CAD build for the part. Positions are in the model's coordinates, mm. Face numbers are marked on the shaded views. Give positions to 0.01 mm unless a question says otherwise; leave off trailing zeros. Loops run counter-clockwise (first coordinate to the right, second up) from the corner with the lowest first, then second, coordinate; pieces in that order, holes last. Notation, with made-up numbers: M -27,-1 L -21,-1 A25 ccw -21,38 Z; hole C -5.5,17.5 d6. An arc over 180 degrees is marked long. Answer as CSV lines item,"result".
```python
from build123d import *

# Parameters (mm, degrees)
F0_R     = 14.235704
F0_R_2   = 10.13824
F1_DEPTH = 50.8
F2_DEPTH = 114.046


with BuildPart() as f1:
    # F0 (on Top) → F1 (new body)
    with BuildSketch(Plane.XY):
        Circle(F0_R)
        with Locations((53.975, 0)):
            Circle(F0_R_2)
        with BuildLine():
            Line((57.191927, 18.776418), (9.512184, 26.945296))
            Line((9.512184, 26.945296), (0, 28.575))
            ThreePointArc((0, 28.575), (-28.575, 0), (0, -28.575))
            Line((0, -28.575), (9.512184, -26.945296))
            Line((9.512184, -26.945296), (57.191927, -18.776418))
            ThreePointArc((57.191927, -18.776418), (73.025, 0), (57.191927, 18.776418))
        make_face()
        Circle(F0_R, mode=Mode.SUBTRACT)
        with Locations((53.975, 0)):
            Circle(F0_R_2, mode=Mode.SUBTRACT)
        with BuildLine():
            Line((0, 28.575), (9.512184, 26.945296))
            ThreePointArc((9.512184, 26.945296), (4.825391, 28.164627), (0, 28.575))
        make_face()
        with BuildLine():
            Line((9.512184, -26.945296), (0, -28.575))
            ThreePointArc((0, -28.575), (4.825391, -28.164627), (9.512184, -26.945296))
        make_face()
    extrude(amount=F1_DEPTH)

    # F0 (on Top) → F2 (cut)
    with BuildSketch(Plane.XY):
        Circle(F0_R)
        with Locations((53.975, 0)):
            Circle(F0_R_2)
    extrude(amount=F2_DEPTH, mode=Mode.SUBTRACT)


solid = f1.part
```
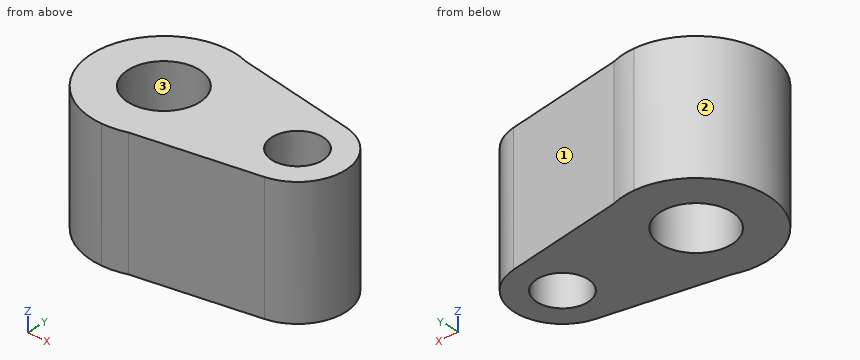
Q1. Cut at B-B (y = 0). Write the cut outline in (x, z) (3 decimals).
Solution:
outline,"M -28.575,0 L -14.236,0 L -14.236,50.8 L -28.575,50.8 Z; M 14.236,0 L 43.837,0 L 43.837,50.8 L 14.236,50.8 Z; M 64.113,0 L 73.025,0 L 73.025,50.8 L 64.113,50.8 Z"
Q2. Cut at C-C (x = -1.5). Write the cut outline in (y, z), and give its area (3 significant figures).
Solution:
outline,"M -28.54,0 L -14.16,0 L -14.16,50.8 L -28.54,50.8 Z; M 14.16,0 L 28.54,0 L 28.54,50.8 L 14.16,50.8 Z"
area,"1,460 mm²"
Q3. Pin check, flat tips, straight feed: P1, Ø1, axis at y = -22, z = 21, coming from the -X side; P2, Ø1, axis at x = -3, z = 45, coming from the +Y side; P3, Ø5, axis at x = 40.5, z = 44, coming from the +Y side; P4, Ø18, axis at x = 53.975, y = 0, coming from the +Z side. Stop position of each tip, or through.
Solution:
P1,"stops at x = -18.82"
P2,"stops at y = 28.47"
P3,"stops at y = 22.06"
P4,"passes through"
Q4. Cut at D-D (x = 61). Write the cut outline in (y, z), and give its area (3 significant figures).
Solution:
outline,"M -17.71,0 L -7.31,0 L -7.31,50.8 L -17.71,50.8 Z; M 7.31,0 L 17.71,0 L 17.71,50.8 L 7.31,50.8 Z"
area,"1,060 mm²"
Q5. Mould opens along X. For the marked faces 1, 2 and 3 say: released by +X, released by -X, zero draft, split by the parting line, or undercut.
Solution:
face 1,"released by +X"
face 2,"released by -X"
face 3,"undercut"
Q6. Wall check: line 1 (X direction, y = 5, z = 17.5); line 2 (Y direction, x = -2, z = 31.5); line 3 (Y direction, x = -7.5, z = 5). Give the ranges that are in metal, low to high. Write a range as [from, to].
Solution:
line 1,"x = [-28.13, -13.33], [13.33, 45.16], [62.79, 72.36]"
line 2,"y = [-28.5, -14.09], [14.09, 28.5]"
line 3,"y = [-27.57, -12.1], [12.1, 27.57]"
Q7. Cut at A-A (z = 38.5). Write the cut outline in (x, y) (3 decimals), and give its area (3 significant figures).
Solution:
outline,"M 0,-28.575 A28.575 ccw 9.512,-26.945 L 57.192,-18.776 A19.05 ccw 57.192,18.776 L 9.512,26.945 A28.575 ccw 0,28.575 A28.575 ccw Z; hole C 0,0 d28.471; hole C 53.975,0 d20.276"
area,"3,480 mm²"
